Read the model definition and answer for the solid it produces. Units are mm, in the model's axes. A direction names the side the tool comes from. Coordinates: 2 decimals unless noted, no trailing zeros. Loops run counter-clockwise (first coordinate to the right, second up) from the corner with the lowest first, then second, coordinate; pieces in that order, holes last. Notation, with made-up numbers: (-34, 64) -> (12, 64) arc R28 cw to (12, 95) -> close; hole circle Ø1 at (10.5, 86). An arc over 180 degrees is marked (long way). Answer in a Markdown table with one row per item.
```python
from build123d import *

# Parameters (mm, degrees)
SKETCH1_W                   = 77
SKETCH1_H                   = 20
BOSS_EXTRUDE1_DEPTH         = 6
TAP_DRILL_FOR_M3_TAP1_D     = 2.5
TAP_DRILL_FOR_M3_TAP1_DEPTH = 10
TAP_DRILL_FOR_M3_TAP1_TIP   = 0.751075774
TAP_DRILL_FOR_M3_TAP2_D     = 2.5
TAP_DRILL_FOR_M3_TAP2_DEPTH = 10
TAP_DRILL_FOR_M3_TAP2_TIP   = 0.751075774
CUT_EXTRUDE1_REACH          = 81.781
SKETCH7_W                   = 10
SKETCH7_H                   = 8
SKETCH7_W_2                 = 49
SKETCH7_H_2                 = 12
FILLET1_R                   = 1.5


with BuildPart() as part:
    # Sketch1 → Boss-Extrude1 (new body)
    with BuildSketch(Plane(origin=(0, 0, 0), x_dir=(1, 0, 0), z_dir=(0, 1, 0))):
        with Locations((38.5, 10)):
            Rectangle(SKETCH1_W, SKETCH1_H)
    extrude(amount=BOSS_EXTRUDE1_DEPTH)

    # Tap Drill for M3 Tap1
    with Locations(Plane.ZY):
        with Locations((-17, 3), (-3, 3)):
            Hole(TAP_DRILL_FOR_M3_TAP1_D / 2, depth=TAP_DRILL_FOR_M3_TAP1_DEPTH)
            with Locations((0, 0, -(TAP_DRILL_FOR_M3_TAP1_DEPTH + TAP_DRILL_FOR_M3_TAP1_TIP / 2))):  # 118° drill point
                Cone(0, TAP_DRILL_FOR_M3_TAP1_D / 2, TAP_DRILL_FOR_M3_TAP1_TIP, mode=Mode.SUBTRACT)

    # Tap Drill for M3 Tap2
    with Locations(Plane(origin=(77, 0, 0), x_dir=(0, 0, -1), z_dir=(1, 0, 0))):
        with Locations((3, 3), (17, 3)):
            Hole(TAP_DRILL_FOR_M3_TAP2_D / 2, depth=TAP_DRILL_FOR_M3_TAP2_DEPTH)
            with Locations((0, 0, -(TAP_DRILL_FOR_M3_TAP2_DEPTH + TAP_DRILL_FOR_M3_TAP2_TIP / 2))):  # 118° drill point
                Cone(0, TAP_DRILL_FOR_M3_TAP2_D / 2, TAP_DRILL_FOR_M3_TAP2_TIP, mode=Mode.SUBTRACT)

    # Sketch7 → Cut-Extrude1 (cut, up to next)
    with BuildSketch(Plane(origin=(0, 6, 0), x_dir=(1, 0, 0), z_dir=(0, 1, 0)), mode=Mode.PRIVATE) as cut_extrude1_sk1:
        with Locations((5, 10)):
            Rectangle(SKETCH7_W, SKETCH7_H)
    cut_extrude1_tool1 = extrude(cut_extrude1_sk1.sketch, amount=-CUT_EXTRUDE1_REACH, mode=Mode.PRIVATE) & part.part
    # Sketch7 → Cut-Extrude1 (cut, up to next)
    with BuildSketch(Plane(origin=(0, 6, 0), x_dir=(1, 0, 0), z_dir=(0, 1, 0)), mode=Mode.PRIVATE) as cut_extrude1_sk2:
        with Locations((38.5, 10)):
            Rectangle(SKETCH7_W_2, SKETCH7_H_2)
    cut_extrude1_tool2 = extrude(cut_extrude1_sk2.sketch, amount=-CUT_EXTRUDE1_REACH, mode=Mode.PRIVATE) & part.part
    # Sketch7 → Cut-Extrude1 (cut, up to next)
    with BuildSketch(Plane(origin=(0, 6, 0), x_dir=(1, 0, 0), z_dir=(0, 1, 0)), mode=Mode.PRIVATE) as cut_extrude1_sk3:
        with Locations((72, 10)):
            Rectangle(SKETCH7_W, SKETCH7_H)
    cut_extrude1_tool3 = extrude(cut_extrude1_sk3.sketch, amount=-CUT_EXTRUDE1_REACH, mode=Mode.PRIVATE) & part.part
    add(cut_extrude1_tool1.solids().sort_by_distance((5, 6, -10))[0], mode=Mode.SUBTRACT)
    add(cut_extrude1_tool2.solids().sort_by_distance((38.5, 6, -10))[0], mode=Mode.SUBTRACT)
    add(cut_extrude1_tool3.solids().sort_by_distance((72, 6, -10))[0], mode=Mode.SUBTRACT)

    # Fillet1
    fillet1_edges = [part.edges().sort_by_distance(p)[0] for p in [
        (10, 3, -14),
        (10, 3, -6),
        (14, 3, -4),
        (14, 3, -16),
        (63, 3, -16),
        (63, 3, -4),
        (67, 3, -6),
        (67, 3, -14),
    ]]
    fillet(fillet1_edges, radius=FILLET1_R)


solid = part.part
```
1. Given pin 1 Ø2 at (y, z) = (3, -3) entering from -X; pin 2 Ø2.5 at (y, z) = (2, -9.5) entering from +X; pin 3 Ø2 at (y, z) = (3, -17) entering from +X, each flat-ended and moving along its own axis, determine where each tip first touches the part or whether it passes through.
A:
| item | result |
|---|---|
| pin 1 | stops at x = 10.15 |
| pin 2 | stops at x = 67 |
| pin 3 | stops at x = 66.85 |
2. A cutting plane is placed at A-A on x = 56. Give the vertices of the cut face in (y, z), and give its area (3 significant figures).
A:
| item | result |
|---|---|
| outline | (0, -20) -> (6, -20) -> (6, -16) -> (0, -16) -> close; (0, -4) -> (6, -4) -> (6, 0) -> (0, 0) -> close |
| area | 48.0 mm2 |
3. The mould has two halves that part along Y. Classify faces 1 (the conical face through (10.62, 2.92, -16.8)), 2 (the flat face through (38, 6, -17)), 3 (the flat face through (0, 3, -15.6)): pulls with the +Y half, pulls with the -Y half, needs draft (parallel to the pull), parting line crosses it, or undercut.
A:
| item | result |
|---|---|
| face 1 | undercut |
| face 2 | pulls with the +Y half |
| face 3 | needs draft |
4. A cutting plane is placed at B-B on y = 0.7. Give the vertices of the cut face in (x, z), and give its area (3 significant figures).
A:
| item | result |
|---|---|
| outline | (0, -20) -> (77, -20) -> (77, -14) -> (68.5, -14) arc R1.5 cw to (67, -12.5) -> (67, -7.5) arc R1.5 cw to (68.5, -6) -> (77, -6) -> (77, 0) -> (0, 0) -> (0, -6) -> (8.5, -6) arc R1.5 cw to (10, -7.5) -> (10, -12.5) arc R1.5 cw to (8.5, -14) -> (0, -14) -> close; hole (14, -14.5) arc R1.5 ccw to (15.5, -16) -> (61.5, -16) arc R1.5 ccw to (63, -14.5) -> (63, -5.5) arc R1.5 ccw to (61.5, -4) -> (15.5, -4) arc R1.5 ccw to (14, -5.5) -> close |
| area | 796 mm2 |
5. Find the intervals of material crossed by probe 1 along Z at (x, y) = (6.5, 3); probe 2 along Z at (x, y) = (4.5, 0.95); probe 3 along X at (y, z) = (0.3, -14.5), in increasing order.
A:
| item | result |
|---|---|
| probe 1 | z = -20 to -18.25, -15.75 to -14, -6 to -4.25, -1.75 to 0 |
| probe 2 | z = -20 to -14, -6 to 0 |
| probe 3 | x = 0 to 14, 63 to 77 |
6. A tool of negligible diameter and unlimited length cuts with its end or side. For faces 4 (the flat face through (63, 3, -10)), 5 (the flat face through (10, 3, -10)), 6 (the flat face through (73, 3, -6)), from which of +Z, -Z, +X, -X, +Y, -Y can it reach the whole face along a straight path? Write none if from no direction.
A:
| item | result |
|---|---|
| face 4 | +Y, -Y |
| face 5 | -X, +Y, -Y |
| face 6 | +X, +Y, -Y |
